Verification items for the finished model (mm, model axes). Face numbers are marked on the shaded views. A direction names the side the tool comes from. Give positions to 0.01 mm unless a question says otherwise; leave off trailing zeros. Order: outer loops, then holes, each group sorted by start corner. A loop starts at its lowest first (then second) coordinate and runs counter-clockwise, first axis right, second up.
from build123d import *

# Parameters (mm, degrees)
SKETCH_W        = 28
SKETCH_H        = 24
SKETCH_R        = 8
PAD_DEPTH       = 5
SKETCH001_R     = 1.6
POCKET_DEPTH    = 24.001
SKETCH002_W     = 28
SKETCH002_H     = 24
PAD001_DEPTH    = 1
SKETCH003_R     = 6.5
POCKET001_DEPTH = 5
FILLET_R        = 1
FILLET001_R     = 1
FILLET002_R     = 1
FILLET003_R     = 1
CHAMFER_SIZE    = 0.4


with BuildPart() as part:
    # Sketch → Pad (new body)
    with BuildSketch(Plane.XY):
        Rectangle(SKETCH_W, SKETCH_H)
        Circle(SKETCH_R, mode=Mode.SUBTRACT)
    extrude(amount=PAD_DEPTH)

    # Sketch001 (on Face3 of Pad) → Pocket (cut, through all)
    with BuildSketch(Plane.XZ.offset(12)):
        with Locations((-10.5, 2)):
            Circle(SKETCH001_R)
        with Locations((10.5, 2)):
            Circle(SKETCH001_R)
    extrude(amount=-POCKET_DEPTH, mode=Mode.SUBTRACT)

    # Sketch002 (on Face3 of Pocket) → Pad001 (join)
    with BuildSketch(Plane(origin=(0, 0, 0), x_dir=(1, 0, 0), z_dir=(0, 0, -1))):
        Rectangle(SKETCH002_W, SKETCH002_H)
    extrude(amount=PAD001_DEPTH)

    # Sketch003 (on Face11 of Pad001) → Pocket001 (cut)
    with BuildSketch(Plane(origin=(0, 0, -1), x_dir=(1, 0, 0), z_dir=(0, 0, -1))):
        Circle(SKETCH003_R)
    extrude(amount=-POCKET001_DEPTH, mode=Mode.SUBTRACT)

    # Fillet
    fillet_edges = [part.edges().sort_by_distance(p)[0] for p in [
        (14, -12, -0.5),
        (14, -12, 2.5),
    ]]
    fillet(fillet_edges, radius=FILLET_R)

    # Fillet001
    fillet001_edges = [part.edges().sort_by_distance(p)[0] for p in [
        (-14, -12, -0.5),
        (-14, -12, 2.5),
    ]]
    fillet(fillet001_edges, radius=FILLET001_R)

    # Fillet002
    fillet002_edges = [part.edges().sort_by_distance(p)[0] for p in [
        (-14, 12, 2.5),
        (-14, 12, -0.5),
    ]]
    fillet(fillet002_edges, radius=FILLET002_R)

    # Fillet003
    fillet003_edges = [part.edges().sort_by_distance(p)[0] for p in [
        (14, 12, 2.5),
        (14, 12, -0.5),
    ]]
    fillet(fillet003_edges, radius=FILLET003_R)

    # Chamfer
    chamfer_edges = [part.edges().sort_by_distance(p)[0] for p in [
        (-8, 0, 5),
    ]]
    chamfer(chamfer_edges, length=CHAMFER_SIZE)


solid = part.part
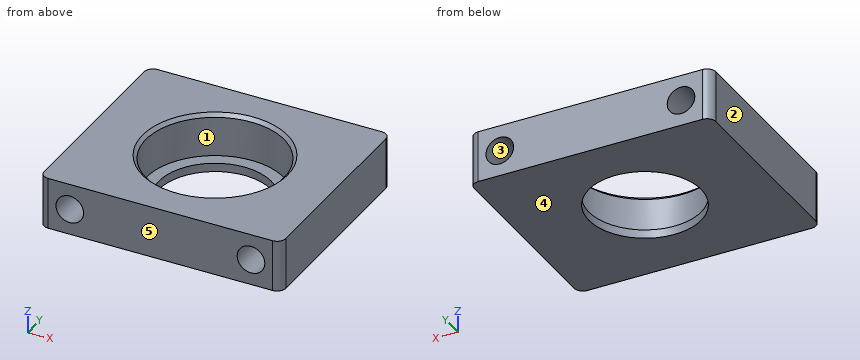
(1) Scan lines: line 1 (X direction, y = -8.25, z = 2.8); line 2 (Y direction, x = 0, z = -0.7); line 3 (X direction, y = 8.75, z = 0.7). Record each from-to range of solid material in increasing order.
Solved:
line 1: x = -14 to -11.89, -9.11 to 9.11, 11.89 to 14
line 2: y = -12 to -6.5, 6.5 to 12
line 3: x = -14 to -11.43, -9.57 to 9.57, 11.43 to 14
(2) Go/stop test with flat-tipped pins: pin 1 (5 mm diameter, centred on x = -5, y = 5, fed in from +Z); pin 2 (5 mm diameter, centred on x = -3.5, y = 3, fed in from +Z); pin 3 (3 mm diameter, centred on x = 10.5, z = 2, fed in from -Y). Record where each tip stops, or that it passes through.
Solved:
pin 1: stops at z = 5
pin 2: stops at z = 0
pin 3: passes through
(3) Section check C-C, the plane z = 2.4. Enter the section's corners in (x, y).
Solved:
outline: (-14, -11) arc R1 ccw to (-13, -12) - (-12.05, -12) - (-12.05, 12) - (-13, 12) arc R1 ccw to (-14, 11) - close; (-8.95, -12) - (8.95, -12) - (8.95, 12) - (-8.95, 12) - close; (12.05, -12) - (13, -12) arc R1 ccw to (14, -11) - (14, 11) arc R1 ccw to (13, 12) - (12.05, 12) - close; hole circle Ø16 at (0, 0)
(4) Set-up check for the marked faces 1 and 2: record each of +Z, -Z, +X, -X, +Y, -Y from which the full face is reachable in a straight line by a thin tool's end or side.
Solved:
face 1: +Z
face 2: +Z, -Z, -X, +Y, -Y
(5) Section check D-D, the plane z = -0.3. Enter the section's corners in (x, y), then the cut area to 3 significant figures.
Solved:
outline: (-14, -11) arc R1 ccw to (-13, -12) - (13, -12) arc R1 ccw to (14, -11) - (14, 11) arc R1 ccw to (13, 12) - (-13, 12) arc R1 ccw to (-14, 11) - close; hole circle Ø13 at (0, 0)
area: 538 mm2
(6) Section check B-B, the plane x = 0. Enter the section's corners in (y, z).
Solved:
outline: (-12, -1) - (-6.5, -1) - (-6.5, 0) - (-8, 0) - (-8, 4.6) - (-8.4, 5) - (-12, 5) - close; (6.5, -1) - (12, -1) - (12, 5) - (8.4, 5) - (8, 4.6) - (8, 0) - (6.5, 0) - close
(7) Release check for a two-part mould opening along Z. For the marked faces 3, 4 and 5 record: pulls with the +Z half, pulls with the -Z half, needs draft (parallel to the pull), parting line crosses it, or undercut.
Solved:
face 3: undercut
face 4: pulls with the -Z half
face 5: needs draft
(8) Section check A-A, the plane y = 0. Enter the section's corners in (x, z).
Solved:
outline: (-14, -1) - (-6.5, -1) - (-6.5, 0) - (-8, 0) - (-8, 4.6) - (-8.4, 5) - (-14, 5) - close; (6.5, -1) - (14, -1) - (14, 5) - (8.4, 5) - (8, 4.6) - (8, 0) - (6.5, 0) - close; hole circle Ø3.2 at (-10.5, 2); hole circle Ø3.2 at (10.5, 2)
